The model under review builds one solid part; all positions refer to its coordinate system, in mm. A direction names the side the tool comes from. Coordinates: 2 decimals unless noted, no trailing zeros. Loops run counter-clockwise (first coordinate to the right, second up) from the corner with the lowest first, then second, coordinate; pieces in that order, holes last. Notation, with made-up numbers: (49.5, 50) -> (108.5, 50) arc R36 ccw to (108.5, 86) -> close; hole circle Ø1 at (0.5, -28). An arc over 180 degrees is marked (long way). One line per question, with ' | ' between items. Start each with the question number.
from build123d import *

# Parameters (mm, degrees)
F1_DEPTH  = 12
F3_DEPTH  = 5
F4_W      = 100
F4_H      = 56
F5_DEPTH  = 2
F6_W      = 130
F6_H      = 5
F7_DEPTH  = 12.001
F9_DEPTH  = 10.001
F11_DEPTH = 5.5
F12_W     = 67
F12_H     = 56
F12_W_2   = 62.5
F12_H_2   = 53
F13_DEPTH = 24
F14_W     = 30
F14_H     = 8
F15_DEPTH = 12.8
F16_W     = 13
F16_H     = 37.5
F17_DEPTH = 2.25
F18_W     = 20
F18_H     = 13
F19_DEPTH = 1.5
F21_D     = 2.7
F21_DEPTH = 12
F21_TIP   = 0.8111618357
F22_W     = 50.5
F22_H     = 38
F23_DEPTH = 2.5
F24_W     = 6.5
F24_H     = 7.5
F24_W_2   = 1
F24_W_3   = 7.5
F25_DEPTH = 24
F27_D     = 2.7
F27_DEPTH = 12
F27_TIP   = 0.8111618357
F28_W     = 5
F28_H     = 17
F29_DEPTH = 2.25
F30_W     = 15
F30_H     = 10
F31_DEPTH = 6
F32_W     = 16
F32_H     = 3
F33_DEPTH = 1


# Not quite as in the source:
# - a feature names something its author has since deleted; it is built from what else it names


with BuildPart() as f1:
    # F0 (on Front) → F1 (new body)
    with BuildSketch(Plane.XZ):
        Polygon((-65, 5), (-65, 0), (65, 0), (65, 5), (50, 5), (50, 61), (-50, 61), (-50, 5), align=None)
    extrude(amount=F1_DEPTH)

    # F2 (on face) → F3 (cut, through all)
    with BuildSketch(Plane(origin=(0, 0, 0), x_dir=(1, 0, 0), z_dir=(0, 0, -1))):
        with BuildLine():
            Line((-65, 2.65), (-63, 2.65))
            ThreePointArc((-63, 2.65), (-59.65, 6), (-63, 9.35))
            Line((-63, 9.35), (-65, 9.35))
            Line((-65, 9.35), (-65, 2.65))
        make_face()
        with BuildLine():
            Line((65, 9.35), (63, 9.35))
            ThreePointArc((63, 9.35), (59.65, 6), (63, 2.65))
            Line((63, 2.65), (65, 2.65))
            Line((65, 2.65), (65, 9.35))
        make_face()
    extrude(amount=-F3_DEPTH, mode=Mode.SUBTRACT)

    # F4 (on face) → F5 (cut)
    with BuildSketch(Plane(origin=(0, 0, 0), x_dir=(-1, 0, 0), z_dir=(0, 1, 0))):
        with Locations((0, 33)):
            Rectangle(F4_W, F4_H)
    extrude(amount=-F5_DEPTH, mode=Mode.SUBTRACT)

    # F6 (on face) → F7 (cut, through all)
    with BuildSketch(Plane(origin=(0, 0, 0), x_dir=(-1, 0, 0), z_dir=(0, 1, 0))):
        with Locations((0, 2.5)):
            Rectangle(F6_W, F6_H)
    extrude(amount=-F7_DEPTH, mode=Mode.SUBTRACT)

    # F8 (on face) → F9 (cut, through all)
    with BuildSketch(Plane.XZ.offset(12)):
        with BuildLine():
            ThreePointArc((-39.5, 34.4), (-36.9, 37), (-39.5, 39.6))
            Line((-39.5, 39.6), (-50, 39.6))
            Line((-50, 39.6), (-50, 34.4))
            Line((-50, 34.4), (-39.5, 34.4))
        make_face()
        with BuildLine():
            Line((-39.5, 19.6), (-50, 19.6))
            Line((-50, 19.6), (-50, 14.4))
            Line((-50, 14.4), (-39.5, 14.4))
            ThreePointArc((-39.5, 14.4), (-36.9, 17), (-39.5, 19.6))
        make_face()
        with BuildLine():
            Line((50, 39.6), (39.5, 39.6))
            ThreePointArc((39.5, 39.6), (36.9, 37), (39.5, 34.4))
            Line((39.5, 34.4), (50, 34.4))
            Line((50, 34.4), (50, 39.6))
        make_face()
        with BuildLine():
            Line((50, 14.4), (50, 19.6))
            Line((50, 19.6), (39.5, 19.6))
            ThreePointArc((39.5, 19.6), (36.9, 17), (39.5, 14.4))
            Line((39.5, 14.4), (50, 14.4))
        make_face()
    extrude(amount=-F9_DEPTH, mode=Mode.SUBTRACT)

    # F10 (on face) → F11 (cut)
    with BuildSketch(Plane.XZ.offset(12)):
        with BuildLine():
            Line((-50, 32.75), (-39.5, 32.75))
            ThreePointArc((-39.5, 32.75), (-35.25, 37), (-39.5, 41.25))
            Line((-39.5, 41.25), (-50, 41.25))
            Line((-50, 41.25), (-50, 39.6))
            Line((-50, 39.6), (-39.5, 39.6))
            ThreePointArc((-39.5, 39.6), (-36.9, 37), (-39.5, 34.4))
            Line((-39.5, 34.4), (-50, 34.4))
            Line((-50, 34.4), (-50, 32.75))
        make_face()
        with BuildLine():
            Line((-39.5, 21.25), (-50, 21.25))
            Line((-50, 21.25), (-50, 19.6))
            Line((-50, 19.6), (-39.5, 19.6))
            ThreePointArc((-39.5, 19.6), (-36.9, 17), (-39.5, 14.4))
            Line((-39.5, 14.4), (-50, 14.4))
            Line((-50, 14.4), (-50, 12.75))
            Line((-50, 12.75), (-39.5, 12.75))
            ThreePointArc((-39.5, 12.75), (-35.25, 17), (-39.5, 21.25))
        make_face()
        with BuildLine():
            Line((50, 39.6), (50, 41.25))
            Line((50, 41.25), (39.5, 41.25))
            ThreePointArc((39.5, 41.25), (35.25, 37), (39.5, 32.75))
            Line((39.5, 32.75), (50, 32.75))
            Line((50, 32.75), (50, 34.4))
            Line((50, 34.4), (39.5, 34.4))
            ThreePointArc((39.5, 34.4), (36.9, 37), (39.5, 39.6))
            Line((39.5, 39.6), (50, 39.6))
        make_face()
        with BuildLine():
            Line((39.5, 12.75), (50, 12.75))
            Line((50, 12.75), (50, 14.4))
            Line((50, 14.4), (39.5, 14.4))
            ThreePointArc((39.5, 14.4), (36.9, 17), (39.5, 19.6))
            Line((39.5, 19.6), (50, 19.6))
            Line((50, 19.6), (50, 21.25))
            Line((50, 21.25), (39.5, 21.25))
            ThreePointArc((39.5, 21.25), (35.25, 17), (39.5, 12.75))
        make_face()
    extrude(amount=-F11_DEPTH, mode=Mode.SUBTRACT)

    # F12 (on face) → F13 (join)
    with BuildSketch(Plane.XZ.offset(12)):
        with Locations((0, 33)):
            Rectangle(F12_W, F12_H)
        with Locations((0, 33)):
            Rectangle(F12_W_2, F12_H_2, mode=Mode.SUBTRACT)
    extrude(amount=F13_DEPTH)

    # F14 (on face) → F15 (join)
    with BuildSketch(Plane.XZ.offset(12)):
        with Locations((-16.25, 10.5)):
            Rectangle(F14_W, F14_H)
    extrude(amount=F15_DEPTH)

    # F16 (on face) → F17 (cut, through all)
    with BuildSketch(Plane(origin=(-33.5, 0, 0), x_dir=(0, -1, 0), z_dir=(-1, 0, 0))):
        with Locations((29.5, 31.25)):
            Rectangle(F16_W, F16_H)
    extrude(amount=-F17_DEPTH, mode=Mode.SUBTRACT)

    # F18 (on face) → F19 (cut, through all)
    with BuildSketch(Plane(origin=(0, 0, 5), x_dir=(1, 0, 0), z_dir=(0, 0, -1))):
        with Locations((17.5, 18.5)):
            Rectangle(F18_W, F18_H)
    extrude(amount=-F19_DEPTH, mode=Mode.SUBTRACT)

    # F21
    with Locations(Plane.XZ.offset(24.8)):
        with Locations((-27.95, 9.5), (-7.95, 9.5)):
            Hole(F21_D / 2, depth=F21_DEPTH)
            with Locations((0, 0, -(F21_DEPTH + F21_TIP / 2))):  # 118° drill point
                Cone(0, F21_D / 2, F21_TIP, mode=Mode.SUBTRACT)

    # F22 (on face) → F23 (cut)
    with BuildSketch(Plane.XZ.offset(12)):
        with Locations((-2, 37.5)):
            Rectangle(F22_W, F22_H)
    extrude(amount=-F23_DEPTH, mode=Mode.SUBTRACT)

    # F24 (on face) → F25 (join, through all)
    with BuildSketch(Plane.XZ.offset(12)):
        with Locations((36.75, 57.25)):
            Rectangle(F24_W, F24_H)
        with Locations((33, 57.25)):
            Rectangle(F24_W_2, F24_H)
        with Locations((36.75, 8.75)):
            Rectangle(F24_W, F24_H)
        with Locations((33, 8.75)):
            Rectangle(F24_W_2, F24_H)
        with Locations((-37.25, 8.75)):
            Rectangle(F24_W_3, F24_H)
        with Locations((-37.25, 57.25)):
            Rectangle(F24_W_3, F24_H)
    extrude(amount=F25_DEPTH)

    # F27
    with Locations(Plane.XZ.offset(36)):
        with Locations((36.25, 57.25), (36.25, 8.75), (-37.25, 8.75), (-37.25, 57.25)):
            Hole(F27_D / 2, depth=F27_DEPTH)
            with Locations((0, 0, -(F27_DEPTH + F27_TIP / 2))):  # 118° drill point
                Cone(0, F27_D / 2, F27_TIP, mode=Mode.SUBTRACT)

    # F28 (on face) → F29 (cut, through all)
    with BuildSketch(Plane.YZ.offset(33.5)):
        with Locations((-33.5, 35.5)):
            Rectangle(F28_W, F28_H)
    extrude(amount=-F29_DEPTH, mode=Mode.SUBTRACT)

    # F30 (on face) → F31 (cut)
    with BuildSketch(Plane(origin=(0, -2, 0), x_dir=(-1, 0, 0), z_dir=(0, 1, 0))):
        with Locations((-42.5, 49)):
            Rectangle(F30_W, F30_H)
    extrude(amount=-F31_DEPTH, mode=Mode.SUBTRACT)

    # F32 (on face) → F33 (cut)
    with BuildSketch(Plane.XZ.offset(24.8)):
        with Locations((-17.95, 13)):
            Rectangle(F32_W, F32_H)
    extrude(amount=-F33_DEPTH, mode=Mode.SUBTRACT)


solid = f1.part
1) Consider section A-A, the plane x = 11.5. Write out the cut boundary in (y, z).
2) Consider section D-D, the plane z = 45.5. Write out the cut boundary in (x, y), plus the area to 4 significant figures.
3) Consider section C-C, the plane y = -21. Write out the cut boundary in (x, z).
4) Wall thickness on L1, parallel to X at y = -32, z = 57; L2, parallel to Z at x = 36, y = -27; L3, parallel to Z at x = -7.95, y = -21.5: over which ranges is each line inside the solid? List them lowest first.
5) Machinability: for faces 4 (the face through (45, -9, 32.75)), 5 (the face through (-32, -23, 31)), 6 (the face through (-45, -4, 34.4)), 7 (the face through (-27.774, -18.716, 10.839)), which of the approach directions +Z, -Z, +X, -X, +Y, -Y give a long, thin tool a straight path to every point of the face, cutting with its end or side? Answer none if there is none.
6) Mouldability with a two-part tool opening along Z and no side actions: class faces 1 (the face through (50, -7, 27)), 2 (the face through (1, -19, 5)), 3 (the face through (-2, -11, 56.5)) as +Z half, -Z half, draft (parallel to the pull), parting line (faces both ways), or undercut.
7) Insertion check: pin 1 Ø4 at (y, z) = (-17, 34.5) entering from -X; pin 2 Ø9 at (y, z) = (-15.5, 11.5) entering from +X; pin 3 Ø1.5 at (x, y) = (26, -15.5) entering from -Z; pin 4 Ø8 at (y, z) = (-28.5, 41.5) entering from -X. Each pin has a flat end and moves straight along its axis. Give the tip position at first contact, or say it passes through.
8) Consider section B-B, the plane y = -32.5. Write out the cut boundary in (x, z).
Filled sheet:
1) outline: (-36, 5) -> (-25, 5) -> (-25, 6.5) -> (-36, 6.5) -> close; (-36, 59.5) -> (-12, 59.5) -> (-12, 56.5) -> (-9.5, 56.5) -> (-9.5, 18.5) -> (-12, 18.5) -> (-12, 5) -> (-2, 5) -> (-2, 61) -> (-36, 61) -> close
2) outline: (-50, -12) -> (-33.5, -12) -> (-33.5, -23) -> (-31.25, -23) -> (-31.25, -12) -> (-27.25, -12) -> (-27.25, -9.5) -> (23.25, -9.5) -> (23.25, -12) -> (31.25, -12) -> (31.25, -36) -> (33.5, -36) -> (33.5, -12) -> (50, -12) -> (50, -8) -> (35, -8) -> (35, -2) -> (-50, -2) -> close | area: 862.5 mm^2
3) outline: (-41, 5) -> (7.5, 5) -> (7.5, 6.5) -> (-1.25, 6.5) -> (-1.25, 14.5) -> (-31.25, 14.5) -> (-31.25, 59.5) -> (31.25, 59.5) -> (31.25, 6.5) -> (27.5, 6.5) -> (27.5, 5) -> (40, 5) -> (40, 12.5) -> (33.5, 12.5) -> (33.5, 53.5) -> (40, 53.5) -> (40, 61) -> (-41, 61) -> (-41, 53.5) -> (-33.5, 53.5) -> (-33.5, 12.5) -> (-41, 12.5) -> close; hole circle Ø2.7 at (-27.95, 9.5); hole circle Ø2.7 at (-7.95, 9.5)
4) L1: -41 to -38.58, -35.92 to -31.25, 31.25 to 34.92, 37.58 to 40 | L2: 5 to 7.42, 10.08 to 12.5, 53.5 to 55.92, 58.58 to 61 | L3: 5 to 8.15, 10.85 to 14.5, 59.5 to 61
5) face 4: +X, -Y | face 5: -X, -Y | face 6: -X, +Y, -Y | face 7: -Y
6) face 1: draft | face 2: -Z half | face 3: undercut
7) pin 1: x = -33.5 | pin 2: x = 50 | pin 3: z = 59.5 | pin 4: x = 31.25
8) outline: (-41, 5) -> (40, 5) -> (40, 12.5) -> (33.5, 12.5) -> (33.5, 27) -> (31.25, 27) -> (31.25, 6.5) -> (-31.25, 6.5) -> (-31.25, 12.5) -> (-41, 12.5) -> close; (-41, 53.5) -> (-33.5, 53.5) -> (-33.5, 50) -> (-31.25, 50) -> (-31.25, 59.5) -> (31.25, 59.5) -> (31.25, 44) -> (33.5, 44) -> (33.5, 53.5) -> (40, 53.5) -> (40, 61) -> (-41, 61) -> close; hole circle Ø2.7 at (-37.25, 8.75); hole circle Ø2.7 at (-37.25, 57.25); hole circle Ø2.7 at (36.25, 8.75); hole circle Ø2.7 at (36.25, 57.25)
